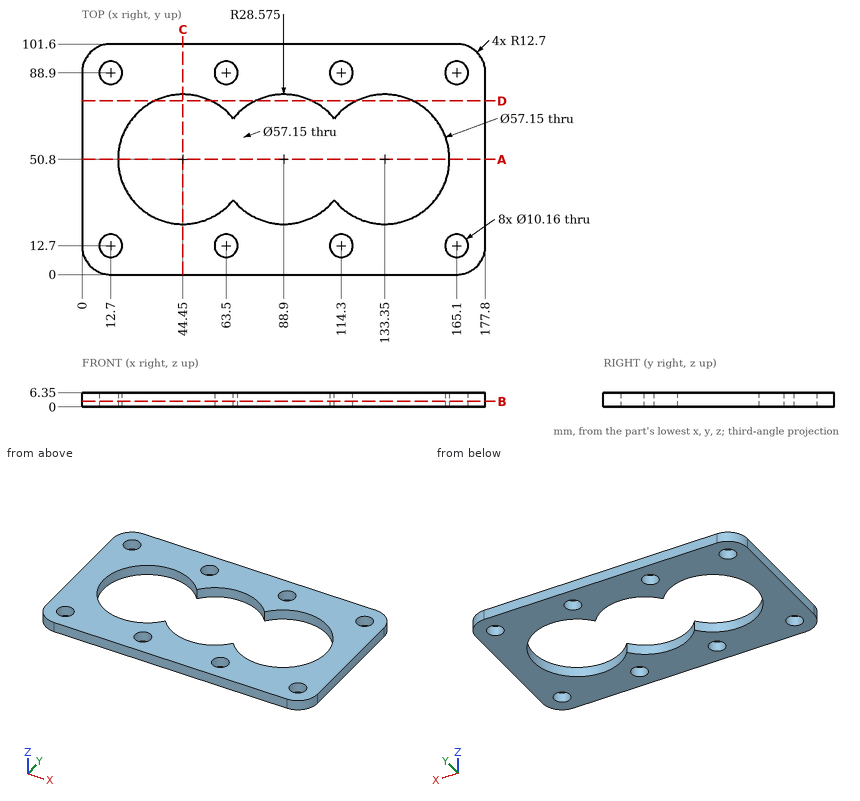
Source: three-view drawing plus pictorial views. Frame: mm from the lowest corner of the part. Round coordinates to 2 decimals unless told otherwise and drop trailing zeros. Loops run counter-clockwise (first coordinate to the right, second up) from the corner with the lowest first, then second, coordinate; pieces in that order, holes last.
Item 1: Section B-B, the plane z = 2.5. State how many separate pieces and enclosed holes the cut face has, plus the area to 3 significant figures.
Checked values:
separate pieces: 1
enclosed holes: 9
area: 10,200 mm2
Item 2: Section D-D, the plane y = 76.5. Output: boundary loops of the cut face in (x, z), plus the area to 3 significant figures.
Checked values:
outline: (0, 0) - (31.96, 0) - (31.96, 6.35) - (0, 6.35) - close; (56.94, 0) - (76.41, 0) - (76.41, 6.35) - (56.94, 6.35) - close; (101.39, 0) - (120.86, 0) - (120.86, 6.35) - (101.39, 6.35) - close; (145.84, 0) - (177.8, 0) - (177.8, 6.35) - (145.84, 6.35) - close
area: 653 mm2
Item 3: Line query: L1, parallel to Y at x = 165.1, z = 3.5; L2, parallel to X at y = 50.8, z = 2.5 (3 decimals); L3, parallel to Y at x = 110, z = 3.75 (3 decimals). Output: solid intervals per line, ascending.
Checked values:
L1: y = 0 to 7.62, 17.78 to 83.82, 93.98 to 101.6
L2: x = 0 to 15.875, 161.925 to 177.8
L3: y = 0 to 9.995, 15.405 to 31.53, 70.07 to 86.195, 91.605 to 101.6
Item 4: Section C-C, the plane x = 44.45. Output: boundary loops of the cut face in (y, z) (3 decimals), plus the area to 3 significant figures.
Checked values:
outline: (0, 0) - (22.225, 0) - (22.225, 6.35) - (0, 6.35) - close; (79.375, 0) - (101.6, 0) - (101.6, 6.35) - (79.375, 6.35) - close
area: 282 mm2
Item 5: Section A-A, the plane y = 50.8. Output: boundary loops of the cut face in (x, z) (3 decimals), plus the area to 3 significant figures.
Checked values:
outline: (0, 0) - (15.875, 0) - (15.875, 6.35) - (0, 6.35) - close; (161.925, 0) - (177.8, 0) - (177.8, 6.35) - (161.925, 6.35) - close
area: 202 mm2
